Source: three-view drawing plus pictorial views. Frame: mm from the lowest corner of the part. A direction names the side the tool comes from. Round coordinates to 2 decimals unless told otherwise and drop trailing zeros. Loops run counter-clockwise (first coordinate to the right, second up) from the corner with the lowest first, then second, coordinate; pieces in that order, holes last. Notation, with made-up numbers: (5, -5.5) -> (62, -5.5) arc R24 cw to (62, 19.5) -> close; hole circle Ø10 at (59, 44.5). An arc over 180 degrees is marked (long way). Answer in a Markdown table with one row per item.
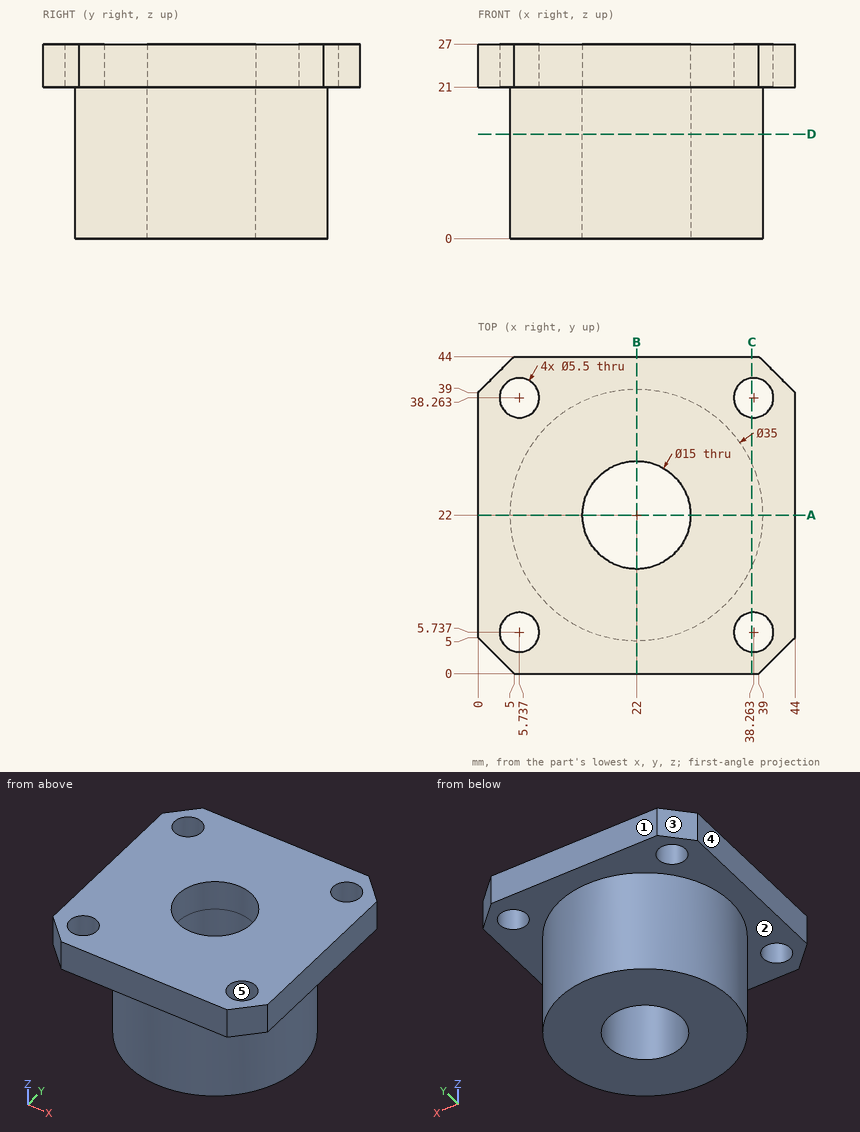
Item 1: Pin query (flat end, axial travel): pin 1 Ø6.5 at (x, y) = (38.26, 38.26) entering from -Z; pin 2 Ø6 at (x, z) = (8.5, 7.5) entering from -Y; pin 3 Ø12 at (x, z) = (25.5, 11.5) entering from -Y; pin 4 Ø12 at (x, y) = (22, 22) entering from +Z. Return the tip coordinate at first contact, or that it passes through.
Answer:
| item | result |
|---|---|
| pin 1 | stops at z = 21 |
| pin 2 | stops at y = 8 |
| pin 3 | stops at y = 4.5 |
| pin 4 | passes through |
Item 2: Cut plane D-D (z = 14.5). Output: boundary loops of the cut face in (x, y).
Answer:
| item | result |
|---|---|
| outline | circle Ø35 at (22, 22); hole circle Ø15 at (22, 22) |
Item 3: Line query: probe 1 along Y at (x, z) = (22, 23.95); probe 2 along X at (y, z) = (5, 24.75) (1 decimal); probe 3 along Y at (x, z) = (16, 11.5). Output: solid intervals per line, ascending. Write a range as [from, to].
Answer:
| item | result |
|---|---|
| probe 1 | y = [0, 14.5], [29.5, 44] |
| probe 2 | x = [0, 3.1], [8.4, 35.6], [40.9, 44] |
| probe 3 | y = [5.56, 17.5], [26.5, 38.44] |
Item 4: Cut plane A-A (y = 22). Output: boundary loops of the cut face in (x, z).
Answer:
| item | result |
|---|---|
| outline | (0, 21) -> (4.5, 21) -> (4.5, 0) -> (14.5, 0) -> (14.5, 27) -> (0, 27) -> close; (29.5, 0) -> (39.5, 0) -> (39.5, 21) -> (44, 21) -> (44, 27) -> (29.5, 27) -> close |
Item 5: Draft query along Y for the marked faces 3, 4 and 5. Return one class per face: pulls with the +Y half, pulls with the -Y half, needs draft (parallel to the pull), parting line crosses it, or undercut.
Answer:
| item | result |
|---|---|
| face 3 | pulls with the +Y half |
| face 4 | needs draft |
| face 5 | undercut |
Item 6: Cut plane C-C (x = 38). Output: boundary loops of the cut face in (y, z).
Answer:
| item | result |
|---|---|
| outline | (0, 21) -> (3, 21) -> (3, 27) -> (0, 27) -> close; (8.47, 21) -> (14.91, 21) -> (14.91, 0) -> (29.09, 0) -> (29.09, 21) -> (35.53, 21) -> (35.53, 27) -> (8.47, 27) -> close; (41, 21) -> (44, 21) -> (44, 27) -> (41, 27) -> close |
Item 7: Reachability of the marked faces 1 and 2 from +Z, -Z, +X, -X, +Y, -Y: full face, straight path, thin tool, end or side. Return the list, or none.
Answer:
| item | result |
|---|---|
| face 1 | +Z, -Z, +X, -X, +Y |
| face 2 | -Z |
